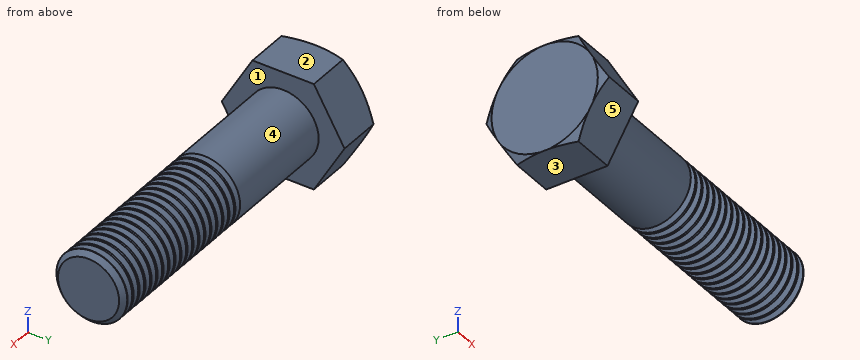
from build123d import *

# Parameters (mm, degrees)
BASEHEAD_DEPTH  = 10.75
THDSCHPAT_COUNT = 19
THDSCHPAT_PITCH = 2


with BuildPart() as part:
    # Sketch1 → BaseHead (new body)
    with BuildSketch(Plane(origin=(0, 0, 0), x_dir=(0, 0, -1), z_dir=(1, 0, 0))):
        Polygon((12, 6.92820323), (12, -6.92820323), (0, -13.856406461), (-12, -6.92820323), (-12, 6.92820323), (0, 13.856406461), align=None)
    extrude(amount=BASEHEAD_DEPTH)

    # BodySke → BaseBody (revolve)
    with BuildSketch(Plane.XY):
        Polygon((0, 0), (75.75, 0), (75.75, 6.8985), (74.6485, 8), (0, 8), align=None)
    revolve(axis=Axis((0, 0, 0), (1, 0, 0)))

    # Sketch3 → HeadChamfer (revolve, cut)
    with BuildSketch(Plane.XY):
        Polygon((0, 12), (3.958548116, 18.856406461), (3.958548116, 23.856406461), (-10, 23.856406461), (-10, 12), align=None)
    revolve(axis=Axis((0, 0, 0), (1, 0, 0)), mode=Mode.SUBTRACT)

    # ThdSchSke → ThreadSchematic (revolve, cut)
    with BuildSketch(Plane.XY):
        Polygon((37.75, -6.8985), (36.978721397, -8), (36.978721397, -10), (38.521278603, -10), (38.521278603, -8), align=None)
    threadschematic = revolve(axis=Axis((-3.175, 0, 0), (1, 0, 0)), mode=Mode.SUBTRACT)

    # ThdSchPat: ThreadSchematic ×19
    with Locations(*[(i * THDSCHPAT_PITCH, 0, 0) for i in range(1, THDSCHPAT_COUNT)]):
        add(threadschematic, mode=Mode.SUBTRACT)


solid = part.part
Can you work these out from the model? Positions are in its coordinate system, mm. Face numbers are marked on the shaded views. A direction names the side the tool comes from. Give positions to 0.01 mm unless a question says otherwise; leave off trailing zeros. Order: outer loops, then holes, each group sorted by start corner. A loop starts at its lowest first (then second) coordinate and runs counter-clockwise, first axis right, second up. Notation, with made-up numbers: (36, -26.5) - (59, -26.5) arc R7 cw to (59, -14.5) - close; hole circle Ø6 at (-3.5, 65). An arc over 180 degrees is marked (long way). Write each question's results on one line, items separated by ' | '.
1) I'm going to push flat-ended pins straight in: pin 1 Ø5 at (x, z) = (53, 8.5) entering from +Y; pin 2 Ø3 at (x, z) = (12.5, 3.5) entering from -Y; pin 3 Ø5 at (x, z) = (65, 9) entering from -Y; pin 4 Ø5 at (x, y) = (68, 11) entering from -Z. Where does each tip first touch, or does it pass through?
Final values:
pin 1: stops at y = 5.29 | pin 2: stops at y = -7.75 | pin 3: stops at y = -4.66 | pin 4: passes through
2) On a 3-axis mill with a long thin cutter (end or side, diameter ignored), from which of +Z, -Z, +X, -X, +Y, -Y can I reach the whole of each face in a straight line? I mean the marked faces 1 and 2. Say none if no direction works.
Final values:
face 1: +X | face 2: +Z, +X, -X, +Y, -Y
3) Suppose I cut it at A-A, the plane x = 26. Write out the boundary of the cut face in (y, z), then the cut area to 3 significant figures.
Final values:
outline: circle Ø16 at (0, 0) | area: 201 mm^2
4) Please list where these lines run through material, in increasing order: line 1 along X through (y, z) = (-9.25, -0.25); line 2 along Z through (x, y) = (21.5, -0.5). Write a range as [from, to].
Final values:
line 1: x = [0, 10.75] | line 2: z = [-7.98, 7.98]
5) If we mould it in two halves opening along Y, with no side actions, what happens to the marked faces 3, 4 and 5? For each: pulls with the +Y half, pulls with the -Y half, needs draft (parallel to the pull), parting line crosses it, or undercut.
Final values:
face 3: needs draft | face 4: parting line crosses it | face 5: pulls with the -Y half
